from build123d import *

# Parameters (mm, degrees)
SKETCH1_R           = 35
SKETCH1_R_2         = 33
BOSS_EXTRUDE1_DEPTH = 30
SKETCH2_W           = 50
SKETCH2_H           = 10
BOSS_EXTRUDE2_DEPTH = 10


with BuildPart() as part:
    # Sketch1 → Boss-Extrude1 (new body)
    with BuildSketch(Plane(origin=(0, 0, 0), x_dir=(1, 0, 0), z_dir=(0, 1, 0))):
        with Locations(Location((0, 0, 0), (0, 0, 270))):
            Circle(SKETCH1_R)
        with Locations(Location((0, 0, 0), (0, 0, 270))):
            Circle(SKETCH1_R_2, mode=Mode.SUBTRACT)
    extrude(amount=BOSS_EXTRUDE1_DEPTH)

    # Sketch2 → Boss-Extrude2 (add)
    with BuildSketch(Plane(origin=(0, 30, 0), x_dir=(1, 0, 0), z_dir=(0, 1, 0))):
        with Locations((-58, 0)):
            Rectangle(SKETCH2_W, SKETCH2_H)
    extrude(amount=-BOSS_EXTRUDE2_DEPTH)


solid = part.part
Input: part model. Units: mm. Frame: model coordinates. A direction names the side the tool comes from. Coordinates: 2 decimals unless noted, no trailing zeros. Loops run counter-clockwise (first coordinate to the right, second up) from the corner with the lowest first, then second, coordinate; pieces in that order, holes last.
Q1. Cut plane C-C (y = 26). Output: boundary loops of the cut face in (x, z).
Q2. Material intervals for line 1 (X direction, y = 24.75, z = 0); line 2 (X direction, y = 18, z = 0); line 3 (Z direction, x = -1, y = 21), sorted ascending.
Q3. Draft query along Z for faces 1 (the face through (-59, 25, -5)), 2 (the face through (-32.215, 14.79, -7.154)), 3 (the face through (-33, 30, -5)). Return one class per face: +Z half, -Z half, draft (parallel to the pull), parting line (faces both ways), or undercut.
Q4. Cut plane D-D (z = -14.5). Output: boundary loops of the cut face in (x, y), then the cut area to 3 significant figures.
Q5. Set-up query: faces 4 (the face through (-59, 20, 0)), 5 (the face through (-59, 25, 5)), 6 (the face through (23.5, 0, -23.5)). Return all of +Z, -Z, +X, -X, +Y, -Y with unobstructed straight access to the full face (end or side cutting, diameter ignored); none if empty.
Q6. Cut plane B-B (x = 0). Output: boundary loops of the cut face in (y, z).
Q7. Cut plane A-A (z = 0). Output: boundary loops of the cut face in (x, y).
Q8. Contact query for flat-ended pins moving along their axis: pin 1 (3 mm diameter, centred on x = -57.5, y = 26, fed in from +Z); pin 2 (5 mm diameter, centred on y = 23, z = 18.5, fed in from -X); pin 3 (1 mm diameter, centred on x = -54.5, y = 26.5, fed in from -Z). Output: stop coordinate, or through.
Working result:
1. outline: (-83, -5) - (-34.64, -5) arc R35 ccw (long way) to (-34.64, 5) - (-83, 5) - close; hole circle Ø66 at (0, 0)
2. line 1: x = -83 to -33, 33 to 35
2. line 2: x = -35 to -33, 33 to 35
2. line 3: z = -34.99 to -32.98, 32.98 to 34.99
3. face 1: -Z half
3. face 2: undercut
3. face 3: draft
4. outline: (-31.86, 0) - (-29.64, 0) - (-29.64, 30) - (-31.86, 30) - close; (29.64, 0) - (31.86, 0) - (31.86, 30) - (29.64, 30) - close
4. area: 133 mm2
5. face 4: +Z, -Z, -X, -Y
5. face 5: +Z, -X, +Y, -Y
5. face 6: +Z, -Z, +X, -X, -Y
6. outline: (0, -35) - (30, -35) - (30, -33) - (0, -33) - close; (0, 33) - (30, 33) - (30, 35) - (0, 35) - close
7. outline: (-83, 20) - (-35, 20) - (-35, 0) - (-33, 0) - (-33, 30) - (-83, 30) - close; (33, 0) - (35, 0) - (35, 30) - (33, 30) - close
8. pin 1: stops at z = 5
8. pin 2: stops at x = -31.13
8. pin 3: stops at z = -5
